from build123d import *

# Parameters (mm, degrees)
BOSS_EXTRUDE1_DEPTH = 1.5
BOSS_EXTRUDE2_DEPTH = 1.5
FILLET1_R           = 1


with BuildPart() as part:
    # Sketch1 → Boss-Extrude1 (new body)
    with BuildSketch(Plane(origin=(0, 0, 0), x_dir=(1, 0, 0), z_dir=(0, 1, 0))):
        Polygon((19.382239382, 38.721878286), (-20.617760618, 38.721878286), (-20.617760618, -26.278121714), (19.382239382, -26.278121714), (19.382239382, -5.478121714), (16.232239382, -5.478121714), (16.232239382, 19.871878286), (19.382239382, 19.871878286), align=None)
    extrude(amount=BOSS_EXTRUDE1_DEPTH)

    # Sketch2 → Boss-Extrude2 (add)
    with BuildSketch(Plane.XZ):
        Polygon((-18.967760618, 24.628121714), (17.732239382, 24.628121714), (17.732239382, 7.128121714), (14.582239382, 7.128121714), (14.582239382, -21.521878286), (17.732239382, -21.521878286), (17.732239382, -37.071878286), (-18.967760618, -37.071878286), align=None)
        Polygon((-17.467760618, 23.128121714), (-17.467760618, -35.571878286), (16.232239382, -35.571878286), (16.232239382, -23.021878286), (13.082239382, -23.021878286), (13.082239382, 8.628121714), (16.232239382, 8.628121714), (16.232239382, 23.128121714), align=None, mode=Mode.SUBTRACT)
    extrude(amount=BOSS_EXTRUDE2_DEPTH)

    # Fillet1
    fillet1_edges = [part.edges().sort_by_distance(p)[0] for p in [
        (19.382239382, 0.75, 26.278121714),
        (-20.617760618, 0.75, 26.278121714),
        (-20.617760618, 0.75, -38.721878286),
        (19.382239382, 0.75, -38.721878286),
    ]]
    fillet(fillet1_edges, radius=FILLET1_R)


solid = part.part
Design review of the part built by this model. Coordinates are the model's own, in mm. A direction names the side the tool comes from. Give positions to 0.01 mm unless a question says otherwise; leave off trailing zeros. Write each loop counter-clockwise with the first axis right and the second up, starting at its lowest first coordinate (ties: lowest second). Pieces come first, ordered by that corner, then holes. Notation, with made-up numbers: M 59.5,9.5 L 67.5,9.5 A23 ccw 67.5,19.5 Z; hole C 59,61 d6. An arc over 180 degrees is marked long. Return JSON: item names as keys, results as strings. Group by question number.
Item 1: Take a section at A-A (y = -0.95). Give the boundary of the cut face in (x, z), plus the area to 3 significant figures.
Item 2: Tool access review of faces 1 (the flat face through (16.232, -1, 16)), 2 (the flat face through (17.732, -1, -29)), 3 (the flat face through (16, -1, -21.522)), 4 (the flat face through (16.232, 1, -7)), 5 (the flat face through (-18.968, -1, -7)): name each direction out of +Z, -Z, +X, -X, +Y, -Y from which nothing blocks a thin tool from reaching the whole face with its end or side.
Item 3: Take a section at C-C (z = -26.5). Give the boundary of the cut face in (x, y), plus the area to 3 significant figures.
Item 4: Take a section at B-B (x = -5). Give the boundary of the cut face in (y, z).
Item 5: Clearance check with flat-ended pins moving along their axes: pin 1 Ø1.6 at (y, z) = (-0.5, -31) entering from +X; pin 2 Ø4 at (x, z) = (9.5, -9.5) entering from -Y; pin 3 Ø1.6 at (y, z) = (-1, -3) entering from +X. State where each tip first meets the part, or that it passes through.
Item 6: Wall thickness on line 1 along X through (y, z) = (-0.65, -25); line 2 along Z through (x, y) = (-15, -1.1); line 3 along Z through (x, y) = (17.5, 0.4): over which ranges is each line inside the solid? List them lowest first.
Item 7: The part is to be moulded in two halves that separate along Z. For faces 6 (the flat face through (14, -1.5, -4)), 7 (the flat face through (-1, -1, 24.628)), 8 (the flat face through (-1, 0, -7)), say which applies: pulls with the +Z half, pulls with the -Z half, needs draft (parallel to the pull), parting line crosses it, or undercut.
Return value:
{
 "1": {"outline": "M -18.97,-37.07 L 17.73,-37.07 L 17.73,-21.52 L 14.58,-21.52 L 14.58,7.13 L 17.73,7.13 L 17.73,24.63 L -18.97,24.63 Z; hole M -17.47,-35.57 L 16.23,-35.57 L 16.23,-23.02 L 13.08,-23.02 L 13.08,8.63 L 16.23,8.63 L 16.23,23.13 L -17.47,23.13 Z", "area": "296 mm2"},
 "2": {"face 1": "-Y", "face 2": "+Z, -Z, +X, -Y", "face 3": "+X, -Y", "face 4": "+X, +Y, -Y", "face 5": "+Z, -Z, -X, -Y"},
 "3": {"outline": "M -20.62,0 L -18.97,0 L -18.97,-1.5 L -17.47,-1.5 L -17.47,0 L 16.23,0 L 16.23,-1.5 L 17.73,-1.5 L 17.73,0 L 19.38,0 L 19.38,1.5 L -20.62,1.5 Z", "area": "64.5 mm2"},
 "4": {"outline": "M -1.5,-37.07 L 0,-37.07 L 0,-38.72 L 1.5,-38.72 L 1.5,26.28 L 0,26.28 L 0,24.63 L -1.5,24.63 L -1.5,23.13 L 0,23.13 L 0,-35.57 L -1.5,-35.57 Z"},
 "5": {"pin 1": "stops at x = 19.38", "pin 2": "stops at y = 0", "pin 3": "stops at x = 14.58"},
 "6": {"line 1": "x = -18.97 to -17.47, 16.23 to 17.73", "line 2": "z = -37.07 to -35.57, 23.13 to 24.63", "line 3": "z = -38.72 to -19.87, 5.48 to 26.28"},
 "7": {"face 6": "needs draft", "face 7": "pulls with the +Z half", "face 8": "undercut"}
}
